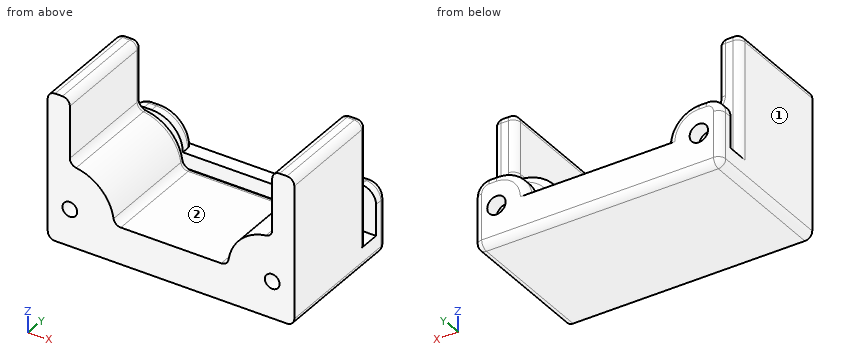
```python
from build123d import *

# Parameters (mm, degrees)
MAIN_BODY_DEPTH                = 15
EXTENSION_FOR_TOP_FLANGE_DEPTH = 2
SKETCH4_R                      = 1.25
TOP_CAMERA_FLANGE_DEPTH        = 2
M2_SCREWHOLE_DEPTH             = 28.028919697
M2_SCREWHOLE_DEPTH_BACK        = 28.028919697
SKETCH5_R                      = 1
FILLET1_R                      = 1


with BuildPart() as part:
    # Sketch2 → Main body (new body)
    with BuildSketch(Plane(origin=(0, 0, 0), x_dir=(1, 0, 0), z_dir=(0, 1, 0))):
        with BuildLine():
            Line((-16.75, -14), (-16.75, 4))
            ThreePointArc((-16.75, 4), (-16.457106781, 4.707106781), (-15.75, 5))
            Line((-15.75, 5), (15.75, 5))
            ThreePointArc((15.75, 5), (16.457106781, 4.707106781), (16.75, 4))
            Line((16.75, 4), (16.75, -14))
            ThreePointArc((16.75, -14), (16.457106781, -14.707106781), (15.75, -15))
            Line((15.75, -15), (14.75, -15))
            ThreePointArc((14.75, -15), (14.042893219, -14.707106781), (13.75, -14))
            Line((13.75, -14), (13.75, -6.92820323))
            ThreePointArc((13.75, -6.92820323), (13.505928946, -6.27354956), (12.892857143, -5.938459912))
            ThreePointArc((12.892857143, -5.938459912), (9.507359313, -4.242640687), (7.811540088, -0.857142857))
            ThreePointArc((7.811540088, -0.857142857), (7.47645044, -0.244071054), (6.82179677, 0))
            Line((6.82179677, 0), (-6.82179677, 0))
            ThreePointArc((-6.82179677, 0), (-7.47645044, -0.244071054), (-7.811540088, -0.857142857))
            ThreePointArc((-7.811540088, -0.857142857), (-9.507359313, -4.242640687), (-12.892857143, -5.938459912))
            ThreePointArc((-12.892857143, -5.938459912), (-13.505928946, -6.27354956), (-13.75, -6.92820323))
            Line((-13.75, -6.92820323), (-13.75, -14))
            ThreePointArc((-13.75, -14), (-14.042893219, -14.707106781), (-14.75, -15))
            Line((-14.75, -15), (-15.75, -15))
            ThreePointArc((-15.75, -15), (-16.457106781, -14.707106781), (-16.75, -14))
        make_face()
    extrude(amount=MAIN_BODY_DEPTH)

    # Sketch3 → Extension for top flange (add)
    with BuildSketch(Plane(origin=(0, 15, 0), x_dir=(1, 0, 0), z_dir=(0, 1, 0))):
        with BuildLine():
            Line((16.75, 2), (16.75, 4))
            ThreePointArc((16.75, 4), (16.457106781, 4.707106781), (15.75, 5))
            Line((15.75, 5), (-15.75, 5))
            ThreePointArc((-15.75, 5), (-16.457106781, 4.707106781), (-16.75, 4))
            Line((-16.75, 4), (-16.75, 2))
            Line((-16.75, 2), (16.75, 2))
        make_face()
    extrude(amount=EXTENSION_FOR_TOP_FLANGE_DEPTH)

    # Sketch4 → Top camera flange (add)
    with BuildSketch(Plane(origin=(0, 17, 0), x_dir=(1, 0, 0), z_dir=(0, 1, 0))):
        with BuildLine():
            Line((16.75, -2.25), (16.75, 2))
            Line((16.75, 2), (16.75, 4))
            ThreePointArc((16.75, 4), (16.457106781, 4.707106781), (15.75, 5))
            Line((15.75, 5), (-15.75, 5))
            ThreePointArc((-15.75, 5), (-16.457106781, 4.707106781), (-16.75, 4))
            Line((-16.75, 4), (-16.75, 2))
            Line((-16.75, 2), (-16.75, -2.25))
            ThreePointArc((-16.75, -2.25), (-16.164213562, -3.664213562), (-14.75, -4.25))
            Line((-14.75, -4.25), (-13.75, -4.25))
            ThreePointArc((-13.75, -4.25), (-10.74479618, -3.00520382), (-9.5, 0))
            Line((-9.5, 0), (9.5, 0))
            ThreePointArc((9.5, 0), (10.74479618, -3.00520382), (13.75, -4.25))
            Line((13.75, -4.25), (14.75, -4.25))
            ThreePointArc((14.75, -4.25), (16.164213562, -3.664213562), (16.75, -2.25))
        make_face()
        with Locations(Location((-13.75, 0, 0), (0, 0, 270))):
            Circle(SKETCH4_R, mode=Mode.SUBTRACT)
        with Locations(Location((13.75, 0, 0), (0, 0, 270))):
            Circle(SKETCH4_R, mode=Mode.SUBTRACT)
    extrude(amount=TOP_CAMERA_FLANGE_DEPTH)

    # Sketch5 → M2 screwhole (cut, two sides: drawn at the far end of the back side and taken through both)
    with BuildSketch(Plane(origin=(0, 15, 0), x_dir=(1, 0, 0), z_dir=(0, 1, 0)).offset(-M2_SCREWHOLE_DEPTH_BACK)):
        with Locations(Location((-13.75, 0, 0), (0, 0, 270))):
            Circle(SKETCH5_R)
        with Locations(Location((13.75, 0, 0), (0, 0, 270))):
            Circle(SKETCH5_R)
    extrude(amount=M2_SCREWHOLE_DEPTH + M2_SCREWHOLE_DEPTH_BACK, mode=Mode.SUBTRACT)

    # Fillet1
    fillet1_edges = [part.edges().sort_by_distance(p)[0] for p in [
        (-13.505928946, 15, 6.27354956),
        (-9.507359313, 15, 4.242640687),
        (-7.47645044, 15, 0.244071054),
        (0, 15, 0),
        (7.47645044, 15, 0.244071054),
        (9.507359313, 15, 4.242640687),
        (13.505928946, 15, 6.27354956),
        (13.75, 15, 10.464101615),
        (14.042893219, 15, 14.707106781),
        (15.25, 15, 15),
        (-14.042893219, 15, 14.707106781),
        (16.457106781, 15, 14.707106781),
        (16.75, 15, 6),
        (-16.75, 15, 6),
        (-16.457106781, 15, 14.707106781),
        (-15.25, 15, 15),
        (16.75, 19, -0.875),
        (16.457106781, 19, -4.707106781),
        (0, 19, -5),
        (-16.457106781, 19, -4.707106781),
        (-16.75, 19, -0.875),
        (-16.164213562, 19, 3.664213562),
        (-14.25, 19, 4.25),
        (-10.74479618, 19, 3.00520382),
        (10.74479618, 19, 3.00520382),
        (14.25, 19, 4.25),
        (16.164213562, 19, 3.664213562),
        (-13.75, 15, 10.464101615),
    ]]
    fillet(fillet1_edges, radius=FILLET1_R)


solid = part.part
```
Model file for the job. Use its own axes, mm. Face numbers are marked on the shaded views. A direction names the side the tool comes from. Round coordinates to 2 decimals unless told otherwise and drop trailing zeros. Write each loop counter-clockwise with the first axis right and the second up, starting at its lowest first coordinate (ties: lowest second). Pieces come first, ordered by that corner, then holes. Notation, with made-up numbers: (-7.5, -6) - (36.5, -6) arc R15 cw to (36.5, 14) - close; hole circle Ø4 at (-37, -10). An arc over 180 degrees is marked (long way). Use CSV: the item, a comma, the result in double quotes. Start each with the question number.
Item 1: Pin check, flat tips, straight feed: P1, Ø1, axis at x = 0, y = 18, coming from the +Z side; P2, Ø1.1, axis at x = -14.5, y = 17.5, coming from the +Z side; P3, Ø0.8, axis at x = 14, y = 17.5, coming from the +Z side; P4, Ø3, axis at x = 6, z = 4, coming from the -Y side. Stop position of each tip, or through.
Item 2: Band-saw the part on D-D (z = 3.75). State how many separate pieces and enclosed holes the cut face has, and give its area (3 significant figures).
Item 3: Band-saw the part on C-C (x = 4.5). Write the cut outline in (y, z), and give its area (3 significant figures).
Item 4: Band-saw the part on B-B (y = 17.5). Write the cut outline in (x, z), and give its area (3 significant figures).
Item 5: Band-saw the part on A-A (z = 10.25). Write the cut outline in (x, y).
Item 6: Drill centre lines: L1, parallel to Y at x = 9, z = -1.25; L2, parallel to Z at x = -1.5, y = 4.75; L3, parallel to X at y = 12.5, z = 4.75. Where is each one in solid material? Low to high. Write a range as [from, to].
Item 7: Tool access for the marked faces 1 and 2: list every direction of +Z, -Z, +X, -X, +Y, -Y with a clear straight run to the whole face (end or side of a thin tool).
Checked values:
1,P1,"stops at z = 0"
1,P2,"stops at z = 4.25"
1,P3,"stops at z = 4.25"
1,P4,"passes through"
2,separate pieces,"4"
2,enclosed holes,"0"
2,area,"245 mm²"
3,outline,"(0, -5) - (18, -5) arc R1 ccw to (19, -4) - (19, 0) - (17, 0) - (17, -2) - (15, -2) - (15, -1) arc R1 ccw to (14, 0) - (0, 0) - close"
3,area,"90.6 mm²"
4,outline,"(-16.75, -4) arc R1 ccw to (-15.75, -5) - (15.75, -5) arc R1 ccw to (16.75, -4) - (16.75, 2.25) arc R2 ccw to (14.75, 4.25) - (13.75, 4.25) arc R4.25 ccw to (9.5, 0) - (-9.5, 0) arc R4.25 ccw to (-13.75, 4.25) - (-14.75, 4.25) arc R2 ccw to (-16.75, 2.25) - close; hole circle Ø2.5 at (-13.75, 0); hole circle Ø2.5 at (13.75, 0)"
4,area,"209 mm²"
5,outline,"(-16.75, 0) - (-13.75, 0) - (-13.75, 14) arc R1 ccw to (-14.75, 15) - (-15.75, 15) arc R1 ccw to (-16.75, 14) - close; (13.75, 0) - (16.75, 0) - (16.75, 14) arc R1 ccw to (15.75, 15) - (14.75, 15) arc R1 ccw to (13.75, 14) - close"
6,L1,"y = [0, 15], [17, 19]"
6,L2,"z = [-5, 0]"
6,L3,"x = [-16.75, -10.08], [10.08, 16.75]"
7,face 1,"+Z, -Z, -X, +Y, -Y"
7,face 2,"+Z, +Y, -Y"
